```python
from build123d import *

# Parameters (mm, degrees)
F1_DEPTH = 15.7734
F2_DEPTH = 40.2336
F3_R     = 3.302


with BuildPart() as f1:
    # F0 (on Top) → F1 (new body)
    with BuildSketch(Plane.XY):
        with BuildLine():
            ThreePointArc((4.370294, 28.238824), (21.695757, 18.596363), (28.575, 0))
            Line((28.575, 0), (33.655, 0))
            ThreePointArc((33.655, 0), (40.750919, 15.428094), (57.082765, 20.080941))
            Line((57.082765, 20.080941), (4.370294, 28.238824))
        make_face()
        with BuildLine():
            Line((33.655, 0), (28.575, 0))
            ThreePointArc((28.575, 0), (21.695757, -18.596363), (4.370294, -28.238824))
            Line((4.370294, -28.238824), (57.082765, -20.080941))
            ThreePointArc((57.082765, -20.080941), (40.750919, -15.428094), (33.655, 0))
        make_face()
        with BuildLine():
            ThreePointArc((57.082765, 20.080941), (40.750919, 15.428094), (33.655, 0))
            ThreePointArc((33.655, 0), (40.750919, -15.428094), (57.082765, -20.080941))
            ThreePointArc((57.082765, -20.080941), (69.403094, -13.224081), (74.295, 0))
            ThreePointArc((74.295, 0), (69.403094, 13.224081), (57.082765, 20.080941))
        make_face()
        with BuildLine():
            ThreePointArc((64.135, 0), (53.975, -10.16), (43.815, 0))
            ThreePointArc((43.815, 0), (53.975, 10.16), (64.135, 0))
        make_face(mode=Mode.SUBTRACT)
    extrude(amount=F1_DEPTH)

    # F0 (on Top) → F2 (join)
    with BuildSketch(Plane.XY):
        with BuildLine():
            ThreePointArc((4.370294, -28.238824), (21.695757, -18.596363), (28.575, 0))
            ThreePointArc((28.575, 0), (21.695757, 18.596363), (4.370294, 28.238824))
            ThreePointArc((4.370294, 28.238824), (-28.575, 0), (4.370294, -28.238824))
        make_face()
        with BuildLine():
            ThreePointArc((13.447765, -4.826), (-14.2875, 0), (13.447765, 4.826))
            Line((13.447765, 4.826), (18.5293, 4.807771))
            Line((18.5293, 4.807771), (18.5293, 0))
            Line((18.5293, 0), (18.5293, -4.807771))
            Line((18.5293, -4.807771), (13.447765, -4.826))
        make_face(mode=Mode.SUBTRACT)
    extrude(amount=F2_DEPTH)

    # F3
    f3_edges = [f1.edges().sort_by_distance(p)[0] for p in [
        (-4.370294, 28.238824, 40.2336),
    ]]
    fillet(f3_edges, radius=F3_R)


solid = f1.part
```
CAD build for the part. Positions are in the model's coordinates, mm. A direction names the side the tool comes from. Coordinates: 2 decimals unless noted, no trailing zeros. Order: outer loops, then holes, each group sorted by start corner. A loop starts at its lowest first (then second) coordinate and runs counter-clockwise, first axis right, second up. Notation, with made-up numbers: (21, 58) - (41, 58) arc R20 cw to (41, 83) - close; hole circle Ø11 at (67.5, -37.75). An arc over 180 degrees is marked (long way). Use a Markdown table: item, result. Add a question column.
(1) Which spindle directions (+Z, -Z, +X, -X, +Y, -Y) get a long thin tool onto all of the face, cutting with end or side? Do faces 4 (the face through (22, 0, 0)), 5 (the face through (18.529, 0, 20)). Say none if no direction does.
(2) Saw through at A-A (x = 58.5). Give the cut face in (y, z), then the cut area to 3 significant figures.
(3) Flat gauge pins, fed straight in: pin 1 (1 mm diameter, centred on x = 18, z = 10.5, fed in from +Y); pin 2 (1 mm diameter, centred on y = -13, z = 34.5, fed in from +X); pin 3 (17 mm diameter, centred on x = 41.5, y = -14, fed in from +Z). Where does each tip first touch, or does it go through?
(4) Drill centre lines: line 1 along X through (y, z) = (-9, 5.5); line 2 along Y through (x, z) = (0, 25) (1 decimal); line 3 along X through (y, z) = (0.5, 16.5). Where is each one in solid material? Low to high. Write a range as [from, to].
(5) Pull direction Y, two halves, no side cores. Call faces 1 (the face through (44.3, 3.1, 7.8)), 2 (the face through (39, 0, 15.773)), 3 (the face through (31.096, 24.103, 7.776)): +Y half, -Y half, draft (parallel to the pull), parting line (faces both ways), or undercut.
Solved:
| question | item | result |
|---|---|---|
| 1 | face 4 | -Z, +X, -X, +Y, -Y |
| 1 | face 5 | +Z, -Z |
| 2 | outline | (-19.81, 0) - (-9.1, 0) - (-9.1, 15.77) - (-19.81, 15.77) - close; (9.1, 0) - (19.81, 0) - (19.81, 15.77) - (9.1, 15.77) - close |
| 2 | area | 338 mm² |
| 3 | pin 1 | stops at y = 26.21 |
| 3 | pin 2 | stops at x = 25.7 |
| 3 | pin 3 | stops at z = 15.77 |
| 4 | line 1 | x = [-27.12, -11.1], [11.1, 49.26], [58.69, 72.19] |
| 4 | line 2 | y = [-28.6, -14.3], [14.3, 28.6] |
| 4 | line 3 | x = [-28.57, -14.28], [18.53, 28.57] |
| 5 | face 1 | undercut |
| 5 | face 2 | draft |
| 5 | face 3 | +Y half |
